Read the model definition and answer for the solid it produces. Units are mm, in the model's axes. A direction names the side the tool comes from. Give positions to 0.01 mm unless a question says otherwise; leave off trailing zeros. Write each loop counter-clockwise with the first axis right and the second up, starting at its lowest first coordinate (ties: lowest second). Pieces come first, ordered by that corner, then holes.
```python
from build123d import *

# Parameters (mm, degrees)
PAD_DEPTH       = 12
POCKET_DEPTH    = 8
POCKET001_DEPTH = 5
PAD001_DEPTH    = 10


with BuildPart() as part:
    # Sketch → Pad (new body)
    with BuildSketch(Plane.XY):
        Polygon((-20.202843, 49.516998), (19.785545, 49.851631), (40, 24.931509), (15.342466, 0.136983), (15.479449, -16.849316), (-15.47945, -16.712328), (-15.47945, -0.273973), (-40.273968, 24.794519), align=None)
    extrude(amount=PAD_DEPTH)

    # Sketch001 (on Face10 of Pad) → Pocket (cut)
    with BuildSketch(Plane.XY.offset(12)):
        Polygon((-12.451404, -1.594348), (-12.451404, -14.745031), (-7.902479, -14.827168), (-8.052838, -1.595545), align=None)
        Polygon((-5.271187, -1.595545), (-5.045653, -14.977527), (-1.061123, -15.052706), (-0.985945, -1.595545), align=None)
        Polygon((1.119081, -1.745904), (1.269447, -15.052706), (5.629864, -14.977527), (5.479505, -1.821082), align=None)
        Polygon((8.411511, -1.896264), (8.250714, -15.208426), (12.696754, -15.127886), (12.922295, -1.971442), align=None)
    extrude(amount=-POCKET_DEPTH, mode=Mode.SUBTRACT)

    # Sketch002 (on Face5 of Pocket) → Pocket001 (cut)
    with BuildSketch(Plane.XY.offset(12)):
        Polygon((-15.068119, 39.735771), (-20.134657, 29.72053), (-8.941154, 29.72053), align=None)
        Polygon((5.315833, 29.83836), (15.920202, 29.83836), (10.264536, 40.324898), align=None)
    extrude(amount=-POCKET001_DEPTH, mode=Mode.SUBTRACT)

    # Sketch003 (on Face5 of Pocket001) → Pad001 (join)
    with BuildSketch(Plane.XY.offset(12)):
        Polygon((-0.533761, 25.884949), (-5.129053, 12.688408), (5.121835, 12.688408), align=None)
    extrude(amount=PAD001_DEPTH)


solid = part.part
```
Item 1: Section A-A (z = 11) is taken. Give the number of separate pieces and of enclosed holes in the cut face, and give its area (3 significant figures).
Result set:
separate pieces: 1
enclosed holes: 6
area: 3,050 mm2
Item 2: Determine the mould class of faces 1 (the flat face through (29.75, 37.57, 5.92)), 2 (the flat face through (-2.8, 19.38, 16.93)), 3 (the flat face through (11, 33, 7)) for opening direction X: pulls with the +X half, pulls with the -X half, needs draft (parallel to the pull), parting line crosses it, or undercut.
Result set:
face 1: pulls with the +X half
face 2: pulls with the -X half
face 3: undercut
Item 3: Section C-C (y = 35.5) is taken. Write down the section's boundary in (x, z).
Result set:
outline: (-31.58, 0) - (31.43, 0) - (31.43, 12) - (12.87, 12) - (12.87, 7) - (7.99, 7) - (7.99, 12) - (-12.48, 12) - (-12.48, 7) - (-17.21, 7) - (-17.21, 12) - (-31.58, 12) - close
Item 4: Which of the six approach directions +Z, -Z, +X, -X, +Y, -Y give full straight-line access (tool end or side, diameter ignored) to faces 4 (the flat face through (0, 24, 0)), 5 (the flat face through (-17.566, 34.798, 9.535)), 6 (the flat face through (0, 12.688, 17))?
Result set:
face 4: -Z, +X, -X, +Y, -Y
face 5: +Z
face 6: +Z, +X, -X, -Y
Item 5: Each of these flat-tipped pins is pushed along its axis until it touches: pin 1 Ø3.5 at (x, y) = (-10.5, -9.5) entering from +Z; pin 2 Ø2 at (y, z) = (4.5, 10.5) entering from -X; pin 3 Ø3 at (x, y) = (11.5, 33.5) entering from +Z; pin 4 Ø3 at (y, z) = (27.5, 17) entering from -X. Where does it stop, or does it pass through?
Result set:
pin 1: stops at z = 4
pin 2: stops at x = -21.19
pin 3: stops at z = 7
pin 4: passes through
Item 6: Find the intervals of material crossed by line 1 along Z through (x, y) = (-3, 42); line 2 along X through (y, z) = (-3.5, 7.75); line 3 along X through (y, z) = (37.5, 8.25), in increasing order.
Result set:
line 1: z = 0 to 12
line 2: x = -15.48 to -12.45, -8.03 to -5.24, -1 to 1.14, 5.5 to 8.39, 12.9 to 15.37
line 3: x = -29.96 to -16.2, -13.7 to 8.93, 11.79 to 29.8
Item 7: Section D-D (x = -17) is taken. Write down the section's boundary in (y, z), and give its area (3 significant figures).
Result set:
outline: (1.26, 0) - (49.54, 0) - (49.54, 12) - (35.92, 12) - (35.92, 7) - (29.72, 7) - (29.72, 12) - (1.26, 12) - close
area: 548 mm2
Item 8: Section B-B (z = 5.5) is taken. Write down the section's boundary in (x, y).
Result set:
outline: (-40.27, 24.79) - (-15.48, -0.27) - (-15.48, -16.71) - (15.48, -16.85) - (15.34, 0.14) - (40, 24.93) - (19.79, 49.85) - (-20.2, 49.52) - close; hole (-12.45, -14.75) - (-7.9, -14.83) - (-8.05, -1.6) - (-12.45, -1.59) - close; hole (-5.27, -1.6) - (-5.05, -14.98) - (-1.06, -15.05) - (-0.99, -1.6) - close; hole (1.12, -1.75) - (1.27, -15.05) - (5.63, -14.98) - (5.48, -1.82) - close; hole (8.25, -15.21) - (12.7, -15.13) - (12.92, -1.97) - (8.41, -1.9) - close
